Design review of the part built by this model. Coordinates are the model's own, in mm. Face numbers are marked on the shaded views. A direction names the side the tool comes from. Coordinates: 2 decimals unless noted, no trailing zeros. Write each loop counter-clockwise with the first axis right and the second up, starting at its lowest first coordinate (ties: lowest second). Pieces come first, ordered by that corner, then holes. Notation, with made-up numbers: (60.25, 49.25) -> (91.25, 49.25) arc R26 ccw to (91.25, 66.25) -> close; hole circle Ø5 at (61.5, 64). An arc over 180 degrees is marked (long way). One line per question, with ' | ' between items. Start each with the question number.
Q1. For P1, Ø1.8, axis at x = 10, y = 4, coming from the +Z side; P2, Ø2.5, axis at x = 6.75, z = 0, coming from the +Y side; P3, Ø3, axis at y = 2.5, z = -3, coming from the -X side, all flat-tipped, find the tip position at first contact; note any pin that passes through.
Q2. Draft analysis for pull direction Z (two halves, no side actions). For the marked faces 1, 2 and 3, state which applies: pulls with the +Z half, pulls with the -Z half, needs draft (parallel to the pull), parting line crosses it, or undercut.
Q3. Wall thickness on probe 1 along X at (y, z) = (1.3, 0); probe 2 along X at (y, z) = (2.3, 0); probe 3 along Y at (x, z) = (-2.5, -1.25): over which ranges is each line inside the solid? List them lowest first.
Q4. Add section D-D on x = -13. State the section outline as (y, z) points, and give its area (3 significant figures).
Q5. Add section C-C on y = 0.45. State the section outline as (x, z) points.
Q6. Add section A-A on y = 2.9. State the section outline as (x, z) points.
Q7. Add section B-B on z = 0. State the section outline as (x, y) points, and give its area (3 significant figures).
Q8. For the marked faces 4, 5, 6, 7 and 8, list the 3-axis set-ups (+Z, -Z, +X, -X, +Y, -Y) from which the entire face can be reached by the end or side of a thin tool; tool diameter is ignored.
from build123d import *

# Parameters (mm, degrees)
SKETCH1_R           = 1.14
SKETCH1_R_2         = 2.05
BOSS_EXTRUDE2_DEPTH = 1.5
SKETCH2_R           = 2.05
BOSS_EXTRUDE3_DEPTH = 4.47
FILLET1_R           = 1.5


with BuildPart() as part:
    # Sketch1 → Boss-Extrude2 (new body)
    with BuildSketch(Plane(origin=(0, 0, 0), x_dir=(1, 0, 0), z_dir=(0, 1, 0))):
        with BuildLine():
            Line((-7.351408028, 3.25), (-14, 3.25))
            ThreePointArc((-14, 3.25), (-17.25, 0), (-14, -3.25))
            Line((-14, -3.25), (-7.351408028, -3.25))
            ThreePointArc((-7.351408028, -3.25), (-5.554548682, -3.578400639), (-3.990008138, -4.521143114))
            ThreePointArc((-3.990008138, -4.521143114), (0, -6.03), (3.990008138, -4.521143114))
            ThreePointArc((3.990008138, -4.521143114), (5.554548682, -3.578400639), (7.351408028, -3.25))
            Line((7.351408028, -3.25), (14, -3.25))
            ThreePointArc((14, -3.25), (17.25, 0), (14, 3.25))
            Line((14, 3.25), (7.351408028, 3.25))
            ThreePointArc((7.351408028, 3.25), (5.554548682, 3.578400639), (3.990008138, 4.521143114))
            ThreePointArc((3.990008138, 4.521143114), (0, 6.03), (-3.990008138, 4.521143114))
            ThreePointArc((-3.990008138, 4.521143114), (-5.554548682, 3.578400639), (-7.351408028, 3.25))
        make_face()
        with Locations(Location((-6.75, 0, 0), (0, 0, 270))):
            Circle(SKETCH1_R, mode=Mode.SUBTRACT)
        with Locations(Location((-14, 0, 0), (0, 0, 270))):
            Circle(SKETCH1_R_2, mode=Mode.SUBTRACT)
        with Locations(Location((6.75, 0, 0), (0, 0, 90))):
            Circle(SKETCH1_R, mode=Mode.SUBTRACT)
        with Locations(Location((14, 0, 0), (0, 0, 90))):
            Circle(SKETCH1_R_2, mode=Mode.SUBTRACT)
    extrude(amount=BOSS_EXTRUDE2_DEPTH)

    # Sketch2 → Boss-Extrude3 (add)
    # profile 1 of 2: a face of its own
    with BuildSketch(Plane(origin=(0, 1.5, 0), x_dir=(1, 0, 0), z_dir=(0, 1, 0))):
        with BuildLine():
            Line((-14, 3.25), (-10, 3.25))
            Line((-10, 3.25), (-10, -3.25))
            Line((-10, -3.25), (-14, -3.25))
            ThreePointArc((-14, -3.25), (-17.25, 0), (-14, 3.25))
        make_face()
        with Locations(Location((-14, 0, 0), (0, 0, 270))):
            Circle(SKETCH2_R, mode=Mode.SUBTRACT)
    # profile 2 of 2: a face of its own
    with BuildSketch(Plane(origin=(0, 1.5, 0), x_dir=(1, 0, 0), z_dir=(0, 1, 0))):
        with BuildLine():
            Line((10, -3.25), (14, -3.25))
            ThreePointArc((14, -3.25), (17.25, 0), (14, 3.25))
            Line((14, 3.25), (10, 3.25))
            Line((10, 3.25), (10, -3.25))
        make_face()
        with Locations(Location((14, 0, 0), (0, 0, 90))):
            Circle(SKETCH2_R, mode=Mode.SUBTRACT)
    extrude(amount=BOSS_EXTRUDE3_DEPTH)

    # Fillet1
    fillet1_edges = [part.edges().sort_by_distance(p)[0] for p in [
        (-10, 3.735, 3.25),
        (-10, 3.735, -3.25),
        (10, 3.735, -3.25),
        (10, 3.735, 3.25),
    ]]
    fillet(fillet1_edges, radius=FILLET1_R)


solid = part.part
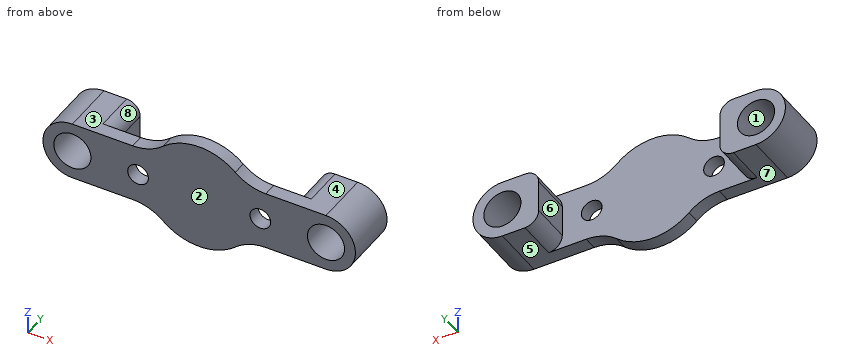
Output values:
1) P1: stops at z = 3.12 | P2: stops at y = 1.5 | P3: stops at x = -16.88
2) face 1: undercut | face 2: needs draft | face 3: pulls with the +Z half
3) probe 1: x = -17.25 to -16.05, -11.95 to -7.89, -5.61 to 5.61, 7.89 to 11.95, 16.05 to 17.25 | probe 2: x = -17.25 to -16.05, -11.95 to -10, 10 to 11.95, 16.05 to 17.25 | probe 3: y = 0 to 1.5
4) outline: (0, -3.25) -> (5.97, -3.25) -> (5.97, -1.79) -> (0, -1.79) -> close; (0, 1.79) -> (5.97, 1.79) -> (5.97, 3.25) -> (0, 3.25) -> close | area: 17.4 mm2
5) outline: (-14, -3.25) -> (-7.35, -3.25) arc R5.08 cw to (-3.99, -4.52) arc R6.03 ccw to (3.99, -4.52) arc R5.08 cw to (7.35, -3.25) -> (14, -3.25) arc R3.25 ccw to (14, 3.25) -> (7.35, 3.25) arc R5.08 cw to (3.99, 4.52) arc R6.03 ccw to (-3.99, 4.52) arc R5.08 cw to (-7.35, 3.25) -> (-14, 3.25) arc R3.25 ccw to start; hole circle Ø4.1 at (-14, 0); hole circle Ø2.28 at (-6.75, 0); hole circle Ø2.28 at (6.75, 0); hole circle Ø4.1 at (14, 0)
6) outline: (-14, -3.25) -> (-11.5, -3.25) arc R1.5 ccw to (-10, -1.75) -> (-10, 1.75) arc R1.5 ccw to (-11.5, 3.25) -> (-14, 3.25) arc R3.25 ccw to start; (10, -1.75) arc R1.5 ccw to (11.5, -3.25) -> (14, -3.25) arc R3.25 ccw to (14, 3.25) -> (11.5, 3.25) arc R1.5 ccw to (10, 1.75) -> close; hole circle Ø4.1 at (-14, 0); hole circle Ø4.1 at (14, 0)
7) outline: (-17.25, 0) -> (-16.05, 0) -> (-16.05, 5.97) -> (-17.25, 5.97) -> close; (-11.95, 0) -> (-7.89, 0) -> (-7.89, 1.5) -> (-10, 1.5) -> (-10, 5.97) -> (-11.95, 5.97) -> close; (-5.61, 0) -> (5.61, 0) -> (5.61, 1.5) -> (-5.61, 1.5) -> close; (7.89, 0) -> (11.95, 0) -> (11.95, 5.97) -> (10, 5.97) -> (10, 1.5) -> (7.89, 1.5) -> close; (16.05, 0) -> (17.25, 0) -> (17.25, 5.97) -> (16.05, 5.97) -> close | area: 60.8 mm2
8) face 4: +Z, +X, +Y, -Y | face 5: -Z, +X, +Y, -Y | face 6: +Z, -Z, +Y | face 7: -Z, -X, +Y, -Y | face 8: +Z, +Y
